Could you check a few things on this model? Use its own coordinates, in mm. A direction names the side the tool comes from. Give positions to 0.01 mm unless a question says otherwise; leave off trailing zeros. Write each loop counter-clockwise with the first axis right and the second up, starting at its lowest first coordinate (ties: lowest second). Pieces come first, ordered by that corner, then holes. Notation, with made-up numbers: (25.25, 1.5) - (52.25, 1.5) arc R20 ccw to (52.25, 35.5) - close; hole circle Ø8 at (-27, -3.75). An arc over 180 degrees is marked (long way). Write item = value, one per line.
from build123d import *

# Parameters (mm, degrees)
SKETCH1_W           = 100
SKETCH1_H           = 60
BOSS_EXTRUDE1_DEPTH = 5
SKETCH2_W           = 5
SKETCH2_H           = 60
BOSS_EXTRUDE2_DEPTH = 57
BOSS_EXTRUDE3_DEPTH = 5
SKETCH5_R           = 35
CUT_EXTRUDE1_DEPTH  = 5


with BuildPart() as part:
    # Sketch1 → Boss-Extrude1 (new body)
    with BuildSketch(Plane(origin=(0, 0, 0), x_dir=(1, 0, 0), z_dir=(0, 1, 0))):
        with Locations((-43.057324841, 0.76433121)):
            Rectangle(SKETCH1_W, SKETCH1_H)
    extrude(amount=BOSS_EXTRUDE1_DEPTH)

    # Sketch2 → Boss-Extrude2 (add)
    with BuildSketch(Plane(origin=(0, 5, 0), x_dir=(1, 0, 0), z_dir=(0, 1, 0))):
        with Locations((4.442675159, 0.76433121)):
            Rectangle(SKETCH2_W, SKETCH2_H)
    extrude(amount=BOSS_EXTRUDE2_DEPTH)

    # Sketch4 → Boss-Extrude3 (add)
    with BuildSketch(Plane(origin=(6.942675159, 0, 0), x_dir=(0, 0, -1), z_dir=(1, 0, 0))):
        Polygon((-29.23566879, 62), (40.76433121, 62), (40.76433121, 142), (-39.23566879, 142), (-39.23566879, 62), align=None)
    extrude(amount=-BOSS_EXTRUDE3_DEPTH)

    # Sketch5 → Cut-Extrude1 (cut)
    with BuildSketch(Plane(origin=(6.942675159, 0, 0), x_dir=(0, 0, -1), z_dir=(1, 0, 0))):
        with Locations((0.76433121, 102)):
            Circle(SKETCH5_R)
    extrude(amount=-CUT_EXTRUDE1_DEPTH, mode=Mode.SUBTRACT)


solid = part.part
1. If we section it at A-A, the plane y = 102: Please give me the cut outline in (x, z), and give its area (3 significant figures).
Filled sheet:
outline = (1.94, -40.76) - (6.94, -40.76) - (6.94, -35.76) - (1.94, -35.76) - close; (1.94, 34.24) - (6.94, 34.24) - (6.94, 39.24) - (1.94, 39.24) - close
area = 50.0 mm2
2. If we section it at B-B, the plane z = -23.5: Please give me the cut outline in (x, y), and give its area (3 significant figures).
Filled sheet:
outline = (-93.06, 0) - (6.94, 0) - (6.94, 75.39) - (1.94, 75.39) - (1.94, 5) - (-93.06, 5) - close; (1.94, 128.61) - (6.94, 128.61) - (6.94, 142) - (1.94, 142) - close
area = 919 mm2
3. Which directions (+Z, -Z, +X, -X, +Y, -Y) give clear straight access to the entire face, cutting with the end or side of a thin tool? Please do faces 5 (the face through (4, 62, 34)), 6 (the face through (4, 62, -36)), 7 (the face through (1.943, 59, 0)), 8 (the face through (-93.057, 2, 0)).
Filled sheet:
face_5 = +Z, +X, -X, -Y
face_6 = -Z, +X, -X, -Y
face_7 = +Z, -Z, -X, +Y
face_8 = +Z, -Z, -X, +Y, -Y
4. If we section it at C-C, the plane y = 133: Please give me the cut outline in (x, z), and give its area (3 significant figures).
Filled sheet:
outline = (1.94, -40.76) - (6.94, -40.76) - (6.94, -17.01) - (1.94, -17.01) - close; (1.94, 15.48) - (6.94, 15.48) - (6.94, 39.24) - (1.94, 39.24) - close
area = 238 mm2
5. I need wall thicknesses on line 1 (X direction, y = 76, z = -36); line 2 (Y direction, x = -75, z = 29). Which ranges of each line are inside material? Lowest first, please.
Filled sheet:
line_1 = 1.94 to 6.94
line_2 = 0 to 5
6. If we section it at D-D, the plane x = -68: Please give me the cut outline in (y, z).
Filled sheet:
outline = (0, -30.76) - (5, -30.76) - (5, 29.24) - (0, 29.24) - close
7. For pin 1 (4 mm diameter, centred on x = 4, z = -36, fed in from -Y); pin 2 (12 mm diameter, centred on y = 28.5, z = 17, fed in from -X); pin 3 (24 mm diameter, centred on y = 101, z = 17, fed in from -X); pin 4 (5 mm diameter, centred on x = -14.5, z = 3, fed in from +Y), each with a flat end and sliding along its axis, tell me the tip position at first contact or that it passes through.
Filled sheet:
pin_1 = 62
pin_2 = 1.94
pin_3 = through
pin_4 = 5
8. Thinking about a two-plate mould opening in Z: for faces 1 (the face through (4.5, 131.5, -19.6)), 2 (the face through (-28, 3, 29.236)), 3 (the face through (4, 101, -40.764)), 4 (the face through (-44, 0, -1)), which applies, pulls with the +Z half, pulls with the -Z half, needs draft (parallel to the pull), parting line crosses it, or undercut?
Filled sheet:
face_1 = undercut
face_2 = pulls with the +Z half
face_3 = pulls with the -Z half
face_4 = needs draft
